Source: CAD feature listing. Evaluate the final solid. Frame: model axes, mm. Face numbers are marked on the shaded views. Coordinates: 2 decimals unless noted, no trailing zeros. Write each loop counter-clockwise with the first axis right and the second up, starting at its lowest first coordinate (ties: lowest second). Pieces come first, ordered by that corner, then holes. Notation, with made-up numbers: (60, 46.25) - (116, 46.25) arc R16 ccw to (116, 70.25) - close; hole circle Ø6 at (89, 20.25). An arc over 180 degrees is marked (long way). One line per item, written item: value.
from build123d import *

# Parameters (mm, degrees)
SKETCH_1_W             = 77.9
SKETCH_1_H             = 47.9
EXTRUDE_1_DEPTH        = 2
SKETCH_2_W             = 47.6
SKETCH_2_H             = 28.6
CUT_EXTRUDE_1_DEPTH    = 27
SKETCH_4_W             = 75.9
SKETCH_4_H             = 45.9
SKETCH_4_W_2           = 47.6
SKETCH_4_H_2           = 28.6
EXTRUDE_3_DEPTH        = 0.5
SKETCH_5_W             = 75.9
SKETCH_5_H             = 45.9
SKETCH_5_W_2           = 47.6
SKETCH_5_H_2           = 28.6
EXTRUDE_4_DEPTH        = 1
SKETCH_8_W             = 3.5
SKETCH_8_H             = 3.5
SKETCH_8_R             = 1
EXTRUDE_5_DEPTH        = 4
FILLET_1_R             = 4
FILLET_1_OF_MIRROR_1_R = 4


with BuildPart() as part:
    # 草图1 → 凸台-拉伸1 (new body)
    with BuildSketch(Plane(origin=(0, 0, 0), x_dir=(1, 0, 0), z_dir=(0, 1, 0))):
        with Locations((38.95, 23.95)):
            Rectangle(SKETCH_1_W, SKETCH_1_H)
    extrude(amount=EXTRUDE_1_DEPTH)

    # 草图2 → 切除-拉伸1 (cut)
    with BuildSketch(Plane(origin=(0, 2, 0), x_dir=(1, 0, 0), z_dir=(0, 1, 0))):
        with Locations((38.95, 23.95)):
            Rectangle(SKETCH_2_W, SKETCH_2_H)
    extrude(amount=-CUT_EXTRUDE_1_DEPTH, mode=Mode.SUBTRACT)

    # 草图4 → 凸台-拉伸3 (add)
    with BuildSketch(Plane.XZ):
        with Locations((38.95, -23.95)):
            Rectangle(SKETCH_4_W, SKETCH_4_H)
        with Locations((38.95, -23.95)):
            Rectangle(SKETCH_4_W_2, SKETCH_4_H_2, mode=Mode.SUBTRACT)
    extrude(amount=EXTRUDE_3_DEPTH)

    # 草图5 → 凸台-拉伸4 (add)
    # profile 1 of 3: a face of its own
    with BuildSketch(Plane.XZ.offset(0.5)):
        with Locations((38.95, -23.95)):
            Rectangle(SKETCH_5_W, SKETCH_5_H)
        with Locations((38.95, -23.95)):
            Rectangle(SKETCH_5_W_2, SKETCH_5_H_2, mode=Mode.SUBTRACT)
    # profile 2 of 3: a face of its own
    with BuildSketch(Plane.XZ.offset(0.5)):
        Polygon((15.15, -38.25), (21.15, -38.25), (21.15, -36.85), (16.55, -36.85), (16.55, -11.05), (21.15, -11.05), (21.15, -9.65), (15.15, -9.65), align=None)
    # profile 3 of 3: a face of its own
    with BuildSketch(Plane.XZ.offset(0.5)):
        Polygon((61.35, -11.05), (61.35, -36.85), (56.75, -36.85), (56.75, -38.25), (62.75, -38.25), (62.75, -9.65), (56.75, -9.65), (56.75, -11.05), align=None)
    extrude(amount=EXTRUDE_4_DEPTH)

    # 草图8 → 凸台-拉伸5 (add)
    # profile 1 of 2: a face of its own
    with BuildSketch(Plane(origin=(76.9, 0, 0), x_dir=(0, 0, -1), z_dir=(1, 0, 0))):
        with Locations((41.15, -3.25)):
            Rectangle(SKETCH_8_W, SKETCH_8_H)
        with Locations((41.15, -3.25)):
            Circle(SKETCH_8_R, mode=Mode.SUBTRACT)
    # profile 2 of 2: a face of its own
    with BuildSketch(Plane(origin=(76.9, 0, 0), x_dir=(0, 0, -1), z_dir=(1, 0, 0))):
        with Locations((15.15, -3.25)):
            Rectangle(SKETCH_8_W, SKETCH_8_H)
        with Locations((15.15, -3.25)):
            Circle(SKETCH_8_R, mode=Mode.SUBTRACT)
    extrude_5 = extrude(amount=-EXTRUDE_5_DEPTH)

    # 圆角1
    # the kernel refuses this fillet: 4 mm, written as the material it adds along each edge
    with BuildSketch(Plane(origin=(76.9, -1.5, -42.9), x_dir=(0, 0, -1), z_dir=(-1, 0, 0)), Plane(origin=(76.9, -1.5, -16.9), x_dir=(0, 0, -1), z_dir=(-1, 0, 0))) as fillet_1_piece_1:
        with BuildLine():
            CenterArc((3.968626967, 4), FILLET_1_R, 187.180755781, 82.819244219)
            Line((0, 3.5), (-0.079372539, 3.49))
            ThreePointArc((-0.079372539, 3.49), (-0.08, 1.75), (-0.08, 0))
            Line((-0.08, 0), (0, -0.08))
            Line((0, -0.08), (3.968626967, -0.08))
            Line((3.968626967, -0.08), (3.968626967, 0))
        make_face()
    extrude(amount=4)
    with BuildSketch(Plane(origin=(76.9, -1.5, -13.4), x_dir=(0, 0, 1), z_dir=(-1, 0, 0)), Plane(origin=(76.9, -1.5, -39.4), x_dir=(0, 0, 1), z_dir=(-1, 0, 0))) as fillet_1_piece_2:
        with BuildLine():
            CenterArc((3.968626967, -4), FILLET_1_R, 90, 82.819244219)
            Line((0, -3.5), (-0.079372539, -3.49))
            ThreePointArc((-0.079372539, -3.49), (-0.08, -1.75), (-0.08, 0))
            Line((-0.08, 0), (0, 0.08))
            Line((0, 0.08), (3.968626967, 0.08))
            Line((3.968626967, 0.08), (3.968626967, 0))
        make_face()
    extrude(amount=4)

    # 镜向1: 凸台-拉伸5 across plane
    add(extrude_5.mirror(Plane(origin=(38.95, 0, 0), x_dir=(0, 0, 1), z_dir=(1, 0, 0))))

    # 圆角1 of 镜向1
    # the kernel refuses this fillet: 4 mm, written as the material it adds along each edge
    with BuildSketch(Plane(origin=(1, -1.5, -42.9), x_dir=(0, 0, -1), z_dir=(1, 0, 0)), Plane(origin=(1, -1.5, -16.9), x_dir=(0, 0, -1), z_dir=(1, 0, 0))) as fillet_1_of_mirror_1_piece_1:
        with BuildLine():
            CenterArc((3.968626967, -4), FILLET_1_OF_MIRROR_1_R, 90, 82.819244219)
            Line((0, -3.5), (-0.079372539, -3.49))
            ThreePointArc((-0.079372539, -3.49), (-0.08, -1.75), (-0.08, 0))
            Line((-0.08, 0), (0, 0.08))
            Line((0, 0.08), (3.968626967, 0.08))
            Line((3.968626967, 0.08), (3.968626967, 0))
        make_face()
    extrude(amount=4)
    with BuildSketch(Plane(origin=(1, -1.5, -13.4), x_dir=(0, 0, 1), z_dir=(1, 0, 0)), Plane(origin=(1, -1.5, -39.4), x_dir=(0, 0, 1), z_dir=(1, 0, 0))) as fillet_1_of_mirror_1_piece_2:
        with BuildLine():
            CenterArc((3.968626967, 4), FILLET_1_OF_MIRROR_1_R, 187.180755781, 82.819244219)
            Line((0, 3.5), (-0.079372539, 3.49))
            ThreePointArc((-0.079372539, 3.49), (-0.08, 1.75), (-0.08, 0))
            Line((-0.08, 0), (0, -0.08))
            Line((0, -0.08), (3.968626967, -0.08))
            Line((3.968626967, -0.08), (3.968626967, 0))
        make_face()
    extrude(amount=4)


solid = part.part
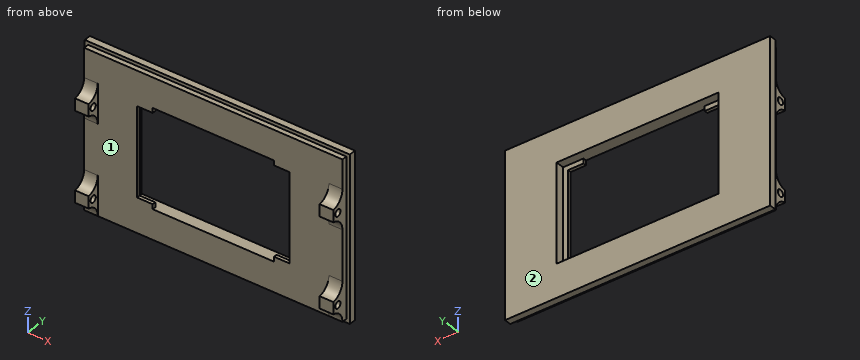
1) Section query D-D on z = -15.15. Output: boundary loops of the cut face in (x, y), then the cut area to 3 significant figures.
Values found:
outline: (0, 0) - (1, 0) - (1, -2.25) - (5, -2.25) - (5, -1.5) - (16.55, -1.5) - (16.55, -0.5) - (15.15, -0.5) - (15.15, 2) - (0, 2) - close; (1, -5) - (5, -5) - (5, -4.25) - (1, -4.25) - close; (61.35, -1.5) - (72.9, -1.5) - (72.9, -2.25) - (76.9, -2.25) - (76.9, 0) - (77.9, 0) - (77.9, 2) - (62.75, 2) - (62.75, -0.5) - (61.35, -0.5) - close; (72.9, -5) - (76.9, -5) - (76.9, -4.25) - (72.9, -4.25) - close
area: 118 mm2
2) Contact query for flat-ended pins moving along their axis: P1, Ø3, axis at y = -4, z = -38.5, coming from the -X side; P2, Ø1, axis at x = 23, z = -38, coming from the -Y side; P3, Ø1.8, axis at y = -3.25, z = -41.15, coming from the +X side; P4, Ø1.1, axis at y = -1, z = -37.5, coming from the +X side. Output: stop coordinate, or through.
Values found:
P1: x = 1
P2: y = -1.5
P3: through
P4: x = 76.9
3) Section query B-B on y = 1. Output: boundary loops of the cut face in (x, z).
Values found:
outline: (0, -47.9) - (77.9, -47.9) - (77.9, 0) - (0, 0) - close; hole (15.15, -38.25) - (62.75, -38.25) - (62.75, -9.65) - (15.15, -9.65) - close
4) Section query A-A on z = -41.15. Output: boundary loops of the cut face in (x, y).
Values found:
outline: (0, 0) - (1, 0) - (1, -2.25) - (5, -2.25) - (5, -1.5) - (72.9, -1.5) - (72.9, -2.25) - (76.9, -2.25) - (76.9, 0) - (77.9, 0) - (77.9, 2) - (0, 2) - close; (1, -5) - (5, -5) - (5, -4.25) - (1, -4.25) - close; (72.9, -5) - (76.9, -5) - (76.9, -4.25) - (72.9, -4.25) - close
5) Section query C-C on x = 24. Output: boundary loops of the cut face in (y, z), then the cut area to 4 significant figures.
Values found:
outline: (-1.5, -46.9) - (0, -46.9) - (0, -47.9) - (2, -47.9) - (2, -38.25) - (-1.5, -38.25) - close; (-1.5, -9.65) - (2, -9.65) - (2, 0) - (0, 0) - (0, -1) - (-1.5, -1) - close
area: 64.55 mm2
6) Material intervals for line 1 (X direction, y = 1.25, z = -29.5); line 2 (Z direction, x = 54.5, y = -1); line 3 (Z direction, x = 16.5, y = 1.5), sorted ascending.
Values found:
line 1: 0 to 15.15, 62.75 to 77.9
line 2: -46.9 to -38.25, -9.65 to -1
line 3: -47.9 to -38.25, -9.65 to 0
7) Draft query along X for the marked faces 1 and 2. Return one class per face: released by +X, released by -X, zero draft, split by the parting line, or undercut.
Values found:
face 1: undercut
face 2: zero draft
